```python
from build123d import *

# Parameters (mm, degrees)
SKETCH_1_W                       = 2
SKETCH_1_H                       = 25
SM_BASE_FLANGE_1_DEPTH           = 22
SM_EDGE_FLANGE_2_STRIP_W         = 9.4732
SM_EDGE_FLANGE_2_STRIP_H         = 2
SM_EDGE_FLANGE_2_STRIP_CUT_DEPTH = 25
SM_EDGE_FLANGE_2_DEPTH           = 25
SKETCH_12_R                      = 3
CUT_EXTRUDE_2_DEPTH              = 10
SKETCH_13_R                      = 2.1
CUT_EXTRUDE_3_DEPTH              = 10
SKETCH_14_W                      = 3.568083007
SKETCH_14_H                      = 26.91386829
CUT_EXTRUDE_4_DEPTH              = 4


# Sheet-metal steps are written as plain solids
with BuildPart() as part:
    # Sketch 1 → 基体-法兰1 (new body)
    with BuildSketch(Plane.XY):
        with Locations((1, 12.5)):
            Rectangle(SKETCH_1_W, SKETCH_1_H)
    extrude(amount=SM_BASE_FLANGE_1_DEPTH)

    # 边线-法兰2 strip (across the edge) → 边线-法兰2 strip cut (cut)
    with BuildSketch(Plane(origin=(2, 25, 22), x_dir=(0, 0, -1), z_dir=(0, -1, 0))):
        with Locations((-2, -1)):
            Rectangle(SM_EDGE_FLANGE_2_STRIP_W, SM_EDGE_FLANGE_2_STRIP_H)
    extrude(amount=SM_EDGE_FLANGE_2_STRIP_CUT_DEPTH, mode=Mode.SUBTRACT)

    # 边线-法兰2 section (across the edge) → 边线-法兰2 (add)
    with BuildSketch(Plane(origin=(2, 25, 22), x_dir=(0, 0, -1), z_dir=(0, -1, 0))):
        with BuildLine():
            Line((0, 0.7366), (0, 13))
            Line((0, 13), (2, 13))
            Line((2, 13), (2, 0.7366))
            ThreePointArc((2, 0.7366), (2.215745145, 0.215745145), (2.7366, 0))
            Line((2.7366, 0), (2.7366, -2))
            ThreePointArc((2.7366, -2), (0.801531583, -1.198468417), (0, 0.7366))
        make_face()
    extrude(amount=SM_EDGE_FLANGE_2_DEPTH)

    # 草图12 → 切除-拉伸2 (cut)
    with BuildSketch(Plane.ZY):
        with Locations((9.13, 4.7)):
            Circle(SKETCH_12_R)
    extrude(amount=-CUT_EXTRUDE_2_DEPTH, mode=Mode.SUBTRACT)

    # 草图13 → 切除-拉伸3 (cut)
    with BuildSketch(Plane(origin=(0, 0, 20), x_dir=(-1, 0, 0), z_dir=(0, 0, -1))):
        with Locations((-9, 13)):
            Circle(SKETCH_13_R)
        with Locations((-9, 22)):
            Circle(SKETCH_13_R)
    extrude(amount=-CUT_EXTRUDE_3_DEPTH, mode=Mode.SUBTRACT)

    # 草图14 → 切除-拉伸4 (cut)
    with BuildSketch(Plane(origin=(0, 0, 0), x_dir=(-1, 0, 0), z_dir=(0, 0, -1))):
        with Locations((-1.784041504, 13.456934145)):
            Rectangle(SKETCH_14_W, SKETCH_14_H)
    extrude(amount=-CUT_EXTRUDE_4_DEPTH, mode=Mode.SUBTRACT)


solid = part.part
```
Part model, mm, in its own coordinate system. A direction names the side the tool comes from. Give positions to 0.01 mm unless a question says otherwise; leave off trailing zeros. Order: outer loops, then holes, each group sorted by start corner. A loop starts at its lowest first (then second) coordinate and runs counter-clockwise, first axis right, second up. Notation, with made-up numbers: (44.25, -39.5) - (51.25, -39.5) arc R19 cw to (51.25, -10.5) - close; hole circle Ø5 at (-0.5, 25.25). An arc over 180 degrees is marked (long way). Use one line per item in the form item = value.
Item 1: Slice it at B-B on z = 9.13. Give the cut face in (x, y), and give its area (3 significant figures).
Solution:
outline = (0, 0) - (2, 0) - (2, 1.7) - (0, 1.7) - close; (0, 7.7) - (2, 7.7) - (2, 25) - (0, 25) - close
area = 38.0 mm2
Item 2: Probe probe 1 along Z at (x, y) = (11, 7); probe 2 along X at (y, z) = (23, 13.75); probe 3 along Z at (x, y) = (1.75, 2.75). List the from-to ranges inside material, lowest first. Write a range as from..to.
Solution:
probe_1 = 20..22
probe_2 = 0..2
probe_3 = 4..6.85, 11.41..21.82
Item 3: Slice it at D-D on z = 5.25. Give the cut face in (x, y).
Solution:
outline = (0, 0) - (2, 0) - (2, 25) - (0, 25) - close
Item 4: Two-plate mould, pull along Y, no slides. Class faces 3 (the face through (0, 12, 12)), 4 (the face through (1, 25, 15)), 5 (the face through (10.548, 23.419, 20.986)), 6 (the face through (11.1, 13.09, 20.99)): released by +Y, released by -Y, zero draft, split by the parting line, or undercut.
Solution:
face_3 = zero draft
face_4 = released by +Y
face_5 = undercut
face_6 = undercut
Item 5: Pin check, flat tips, straight feed: pin 1 Ø3.5 at (x, y) = (10, 11) entering from -Z; pin 2 Ø1.5 at (x, z) = (6, 19) entering from +Y; pin 3 Ø3 at (y, z) = (21.5, 6.5) entering from +X. Stop position of each tip, or through.
Solution:
pin_1 = 20
pin_2 = through
pin_3 = 2
Item 6: Which spindle directions (+Z, -Z, +X, -X, +Y, -Y) get a long thin tool onto all of the face, cutting with end or side? Do faces 1 (the face through (1, 13, 4)), 2 (the face through (9, 10, 20)). Say none if no direction does.
Solution:
face_1 = -Z, +X, -X, +Y, -Y
face_2 = -Z, +X, +Y, -Y
Item 7: Slice it at C-C on y = 13. Give the cut face in (x, z).
Solution:
outline = (0, 4) - (2, 4) - (2, 19.26) arc R0.74 cw to (2.74, 20) - (6.9, 20) - (6.9, 22) - (2.74, 22) arc R2.74 ccw to (0, 19.26) - close; (11.1, 20) - (15, 20) - (15, 22) - (11.1, 22) - close
Item 8: Slice it at A-A on y = 4.7. Give the cut face in (x, z), and give its area (3 significant figures).
Solution:
outline = (0, 4) - (2, 4) - (2, 6.13) - (0, 6.13) - close; (0, 12.13) - (2, 12.13) - (2, 19.26) arc R0.74 cw to (2.74, 20) - (15, 20) - (15, 22) - (2.74, 22) arc R2.74 ccw to (0, 19.26) - close
area = 48.5 mm2
